Geometry: final body of the model. Coordinates: model frame, mm. A direction names the side the tool comes from. Give positions to 0.01 mm unless a question says otherwise; leave off trailing zeros. Order: outer loops, then holes, each group sorted by start corner. A loop starts at its lowest first (then second) coordinate and runs counter-clockwise, first axis right, second up. Notation, with made-up numbers: (73.25, 4) - (91.25, 4) arc R27 ccw to (91.25, 29) - close; hole circle Ø10 at (71.5, -38). An arc over 180 degrees is marked (long way). Put each result on its own line as item: value. Start each with the question number.
1. Section B-B on y = -1. Return the cut outline in (x, z).
2. Set-up query: faces 1 (the flat face through (0, -26, 15)), 2 (the flat face through (55.7, -26.8, 21.4)). Return all of +Z, -Z, +X, -X, +Y, -Y with unobstructed straight access to the full face (end or side cutting, diameter ignored); none if empty.
3. Section D-D on y = 17.5. Return the cut outline in (x, z).
4. Section A-A on x = 63. Return the cut outline in (y, z).
5. First-contact query: P1, Ø0.8, axis at y = 27, z = 16.5, coming from the -X side; P2, Ø7, axis at x = -26, z = 20, coming from the +Y side; P3, Ø5, axis at x = 0, y = -17.5, coming from the +Z side; P4, Ø2, axis at x = -73.5, z = 15, coming from the +Y side. Flat tips, straight axial feed; report the tip coordinate or a pass-through.
6. Ray query, line 1 along Y through (x, z) = (0, 27.6); line 2 along Z through (x, y) = (56, 23); line 3 along X through (y, z) = (-12, 6.5). Return the intervals inside material, ascending. Write a range as from..to.
7. Mould query, pull axis X, two halves, no side actions, for faces 3 (the flat face through (-74, -2, 14)), 4 (the cylindrical face through (73.14, -0.38, 25.6)). Classes: pulls with the +X half, pulls with the -X half, needs draft (parallel to the pull), parting line crosses it, or undercut.
8. Section C-C on x = -39.5. Return the cut outline in (y, z).
from build123d import *

# Parameters (mm, degrees)
ESBO_O1_W                = 155
ESBO_O1_H                = 55
RESSALTO_EXTRUS_O1_DEPTH = 28
ESBO_O3_W                = 148
ESBO_O3_H                = 25
CORTE_EXTRUS_O1_DEPTH    = 100.071943556
CORTE_EXTRUS_O2_REACH    = 161.891
RESSALTO_EXTRUS_O2_REACH = 158.501
ESBO_O6_W                = 2
ESBO_O6_H                = 1.5
RESSALTO_EXTRUS_O3_REACH = 158.501
ESBO_O7_W                = 2
ESBO_O7_H                = 1.5
ESBO_O9_W                = 21
ESBO_O9_H                = 1.5
RESSALTO_EXTRUS_O4_DEPTH = 1.5
FILETE1_R                = 5
FILETE2_R                = 3
RESSALTO_EXTRUS_O5_DEPTH = 1.5
CORTE_EXTRUS_O5_REACH    = 88.871
ESBO_O15_R               = 2


with BuildPart() as part:
    # Esboço1 → Ressalto-extrusão1 (new body)
    with BuildSketch(Plane.XY):
        Rectangle(ESBO_O1_W, ESBO_O1_H)
    extrude(amount=RESSALTO_EXTRUS_O1_DEPTH)

    # Esboço3 → Corte-extrusão1 (cut, through all)
    with BuildSketch(Plane.XZ.offset(27.5)):
        with Locations((0, 14)):
            Rectangle(ESBO_O3_W, ESBO_O3_H)
    extrude(amount=-CORTE_EXTRUS_O1_DEPTH, mode=Mode.SUBTRACT)

    # Esboço4 → Corte-extrusão2 (cut, up to next)
    with BuildSketch(Plane.ZY.offset(77.5), mode=Mode.PRIVATE) as corte_extrus_o2_sk1:
        Polygon((3.5, 27.5), (3.5, 26), (1.5, 26), (1.5, 23.9), (26.5, 23.9), (26.5, 26), (24.5, 26), (24.5, 27.5), align=None)
    corte_extrus_o2_tool1 = extrude(corte_extrus_o2_sk1.sketch, amount=-CORTE_EXTRUS_O2_REACH, mode=Mode.PRIVATE) & part.part
    add(corte_extrus_o2_tool1.solids().sort_by_distance((-77.5, 25.625, 14))[0], mode=Mode.SUBTRACT)

    # Esboço6 → Ressalto-extrusão2 (add, up to next)
    with BuildSketch(Plane(origin=(-74, 0, 0), x_dir=(0, 0, -1), z_dir=(1, 0, 0)), mode=Mode.PRIVATE) as ressalto_extrus_o2_sk1:
        with Locations((-2.5, 26.75)):
            Rectangle(ESBO_O6_W, ESBO_O6_H)
    ressalto_extrus_o2_tool1 = extrude(ressalto_extrus_o2_sk1.sketch, amount=RESSALTO_EXTRUS_O2_REACH, mode=Mode.PRIVATE) - part.part
    add(ressalto_extrus_o2_tool1.solids().sort_by_distance((-74, 26.75, 2.5))[0])

    # Esboço7 → Ressalto-extrusão3 (add, up to next)
    with BuildSketch(Plane(origin=(-74, 0, 0), x_dir=(0, 0, -1), z_dir=(1, 0, 0)), mode=Mode.PRIVATE) as ressalto_extrus_o3_sk1:
        with Locations((-25.5, 26.75)):
            Rectangle(ESBO_O7_W, ESBO_O7_H)
    ressalto_extrus_o3_tool1 = extrude(ressalto_extrus_o3_sk1.sketch, amount=RESSALTO_EXTRUS_O3_REACH, mode=Mode.PRIVATE) - part.part
    add(ressalto_extrus_o3_tool1.solids().sort_by_distance((-74, 26.75, 25.5))[0])

    # Esboço9 → Ressalto-extrusão4 (add)
    with BuildSketch(Plane.ZY.offset(-74)):
        with Locations((14, 26.75)):
            Rectangle(ESBO_O9_W, ESBO_O9_H)
    extrude(amount=RESSALTO_EXTRUS_O4_DEPTH)

    # Filete1
    filete1_edges = [part.edges().sort_by_distance(p)[0] for p in [
        (-77.5, 0, 28),
        (-77.5, 0, 0),
        (77.5, 0, 0),
        (77.5, 0, 28),
    ]]
    fillet(filete1_edges, radius=FILETE1_R)

    # Filete2
    filete2_edges = [part.edges().sort_by_distance(p)[0] for p in [
        (-74, -1.8, 26.5),
        (-74, -1.8, 1.5),
        (74, -0.75, 1.5),
        (74, -0.75, 26.5),
    ]]
    fillet(filete2_edges, radius=FILETE2_R)

    # Esboço12 → Ressalto-extrusão5 (add)
    with BuildSketch(Plane.XZ.offset(27.5)):
        Polygon((-21.304721722, 26.5), (-17.559412156, 26.5), (-27.546904334, 14), (-17.559412156, 1.5), (-21.304721722, 1.5), (-29.419559117, 11.65625), (-37.534396511, 1.5), (-41.279706078, 1.5), (-31.2922139, 14), (-41.279706078, 26.5), (-37.534396511, 26.5), (-29.419559117, 16.34375), align=None)
        Polygon((-71, 26.5), (-61.012507822, 14), (-71, 1.5), (-67.254690433, 1.5), (-59.139853039, 11.65625), (-51.025015645, 1.5), (-47.279706078, 1.5), (-57.267198256, 14), (-47.279706078, 26.5), (-51.025015645, 26.5), (-59.139853039, 16.34375), (-67.254690433, 26.5), align=None)
        Polygon((0.300734805, 16.34375), (-7.814102589, 26.5), (-11.559412156, 26.5), (-1.571919978, 14), (-11.559412156, 1.5), (-7.814102589, 1.5), (0.300734805, 11.65625), (8.4155722, 1.5), (12.160881766, 1.5), (2.173389589, 14), (12.160881766, 26.5), (8.4155722, 26.5), align=None)
        Polygon((30.021028727, 16.34375), (21.906191333, 26.5), (18.160881766, 26.5), (28.148373944, 14), (18.160881766, 1.5), (21.906191333, 1.5), (30.021028727, 11.65625), (38.135866122, 1.5), (41.881175688, 1.5), (31.893683511, 14), (41.881175688, 26.5), (38.135866122, 26.5), align=None)
        Polygon((59.741322649, 16.34375), (51.626485255, 26.5), (47.881175688, 26.5), (57.868667866, 14), (47.881175688, 1.5), (51.626485255, 1.5), (59.741322649, 11.65625), (67.856160044, 1.5), (71.60146961, 1.5), (61.613977433, 14), (71.60146961, 26.5), (67.856160044, 26.5), align=None)
    extrude(amount=-RESSALTO_EXTRUS_O5_DEPTH)

    # Esboço15 → Corte-extrusão5 (cut, up to next)
    with BuildSketch(Plane.XY.offset(28), mode=Mode.PRIVATE) as corte_extrus_o5_sk1:
        with Locations((0, 17.5)):
            Circle(ESBO_O15_R)
    corte_extrus_o5_tool1 = extrude(corte_extrus_o5_sk1.sketch, amount=-CORTE_EXTRUS_O5_REACH, mode=Mode.PRIVATE) & part.part
    # Esboço15 → Corte-extrusão5 (cut, up to next)
    with BuildSketch(Plane.XY.offset(28), mode=Mode.PRIVATE) as corte_extrus_o5_sk2:
        with Locations((0, -17.5)):
            Circle(ESBO_O15_R)
    corte_extrus_o5_tool2 = extrude(corte_extrus_o5_sk2.sketch, amount=-CORTE_EXTRUS_O5_REACH, mode=Mode.PRIVATE) & part.part
    add(corte_extrus_o5_tool1.solids().sort_by_distance((0, 17.5, 28))[0], mode=Mode.SUBTRACT)
    add(corte_extrus_o5_tool2.solids().sort_by_distance((0, -17.5, 28))[0], mode=Mode.SUBTRACT)


solid = part.part
Resolved:
1. outline: (-77.5, 5) arc R5 ccw to (-72.5, 0) - (72.5, 0) arc R5 ccw to (77.5, 5) - (77.5, 23) arc R5 ccw to (72.5, 28) - (-72.5, 28) arc R5 ccw to (-77.5, 23) - close; hole (-74, 4.5) arc R3 ccw to (-71, 1.5) - (71, 1.5) arc R3 ccw to (74, 4.5) - (74, 23.5) arc R3 ccw to (71, 26.5) - (-71, 26.5) arc R3 ccw to (-74, 23.5) - close
2. face 1: none
2. face 2: -Y
3. outline: (-77.5, 5) arc R5 ccw to (-72.5, 0) - (72.5, 0) arc R5 ccw to (77.5, 5) - (77.5, 23) arc R5 ccw to (72.5, 28) - (2, 28) - (2, 26.5) - (71, 26.5) arc R3 cw to (74, 23.5) - (74, 4.5) arc R3 cw to (71, 1.5) - (-71, 1.5) arc R3 cw to (-74, 4.5) - (-74, 23.5) arc R3 cw to (-71, 26.5) - (-2, 26.5) - (-2, 28) - (-72.5, 28) arc R5 ccw to (-77.5, 23) - close
4. outline: (-27.5, 0) - (27.5, 0) - (27.5, 3.5) - (26, 3.5) - (26, 1.5) - (-27.5, 1.5) - close; (-27.5, 7.58) - (-26, 7.58) - (-26, 12.27) - (-27.5, 12.27) - close; (-27.5, 15.73) - (-26, 15.73) - (-26, 20.42) - (-27.5, 20.42) - close; (-27.5, 26.5) - (26, 26.5) - (26, 24.5) - (27.5, 24.5) - (27.5, 28) - (-27.5, 28) - close
5. P1: x = 72.5
5. P2: y = -26
5. P3: z = 28
5. P4: y = 23.9
6. line 1: -27.5..-19.5, -15.5..15.5, 19.5..27.5
6. line 2: 0..1.5, 26.5..28
6. line 3: -77.5..-74, 74..77.5
7. face 3: undercut
7. face 4: undercut
8. outline: (-27.5, 0) - (27.5, 0) - (27.5, 3.5) - (26, 3.5) - (26, 1.5) - (-26, 1.5) - (-26, 3.73) - (-27.5, 3.73) - close; (-27.5, 24.27) - (-26, 24.27) - (-26, 26.5) - (26, 26.5) - (26, 24.5) - (27.5, 24.5) - (27.5, 28) - (-27.5, 28) - close
